Read the model definition and answer for the solid it produces. Units are mm, in the model's axes. A direction names the side the tool comes from. Coordinates: 2 decimals unless noted, no trailing zeros. Write each loop counter-clockwise with the first axis right and the second up, starting at its lowest first coordinate (ties: lowest second). Pieces come first, ordered by that corner, then holes. Notation, with made-up numbers: (88.25, 60) -> (97.25, 60) arc R11 cw to (97.25, 81) -> close; hole circle Ø8 at (78, -3). An arc over 180 degrees is marked (long way). Answer in a Markdown table with one row per item. Add a question column.
Item 1: Which of the six approach directions +Z, -Z, +X, -X, +Y, -Y give full straight-line access (tool end or side, diameter ignored) to faces 1 (the face through (19, 1, -11)), 2 (the face through (-12, 1, 19)), 3 (the face through (-12, 1, -19)), 4 (the face through (19, 1, 12)), 5 (the face through (2, 7, 46))?
Item 2: For a pull along X with two mould halves and no side action, classify faces 6 (the face through (4, 1, 34)), 7 (the face through (48, 11, 0)), 8 (the face through (44.391, 7.056, -0.028)), 9 (the face through (-4, 1, -34)) as +X half, -X half, draft (parallel to the pull), parting line (faces both ways), or undercut.
Item 3: Section C-C on y = 6.5 is taken. Count the separate pieces of the cut face and the enclosed holes in it, then the cut area to 3 significant figures.
Item 4: Straight lines are drawn through the part: line 1 (Z direction, x = -48, y = 2); line 2 (Y direction, x = 10, z = -17). For each, find the intervals that lie inside material, in ascending order. Write a range as from..to.
Item 5: Section A-A on x = 27.5 is taken. Write down the section's boundary in (y, z).
Item 6: Given pin 1 Ø12 at (x, z) = (0.5, -26) entering from +Y; pin 2 Ø1.1 at (x, y) = (48.5, 4) entering from +Z; pin 3 Ø1.1 at (y, z) = (4, -48.5) entering from +X; pin 4 Ø12 at (x, z) = (21, 25.5) entering from -Y, each flat-ended and moving along its own axis, determine where each tip first touches the part or whether it passes through.
Item 7: Section B-B on z = 16 is taken. Write down the section's boundary in (x, y).
```python
from build123d import *

# Parameters (mm, degrees)
SKETCH1_W           = 38
SKETCH1_H           = 38
BOSS_EXTRUDE1_DEPTH = 3
SKETCH2_W           = 30
SKETCH2_H           = 8
BOSS_EXTRUDE2_DEPTH = 3
SKETCH8_R           = 2.5
BOSS_EXTRUDE5_DEPTH = 2
CIRPATTERN1_COUNT   = 4


with BuildPart() as part:
    # Sketch1 → Boss-Extrude1 (new body)
    with BuildSketch(Plane(origin=(0, 0, 0), x_dir=(1, 0, 0), z_dir=(0, 1, 0))):
        Rectangle(SKETCH1_W, SKETCH1_H)
    extrude(amount=BOSS_EXTRUDE1_DEPTH)

    # Sketch2 → Boss-Extrude2 (add)
    with BuildSketch(Plane(origin=(0, 0, 0), x_dir=(1, 0, 0), z_dir=(0, 1, 0))):
        with Locations((-34, 0)):
            Rectangle(SKETCH2_W, SKETCH2_H)
    boss_extrude2 = extrude(amount=BOSS_EXTRUDE2_DEPTH)

    # Sweep1: sweep along a path in Sketch7
    with BuildLine(Plane.XY) as sweep1_path:
        Line((-46.5, 3), (-58.047005384, 23))
    # Sketch8 → Sweep1 (sweep)
    with BuildSketch(Plane(origin=(0, 3, 0), x_dir=(1, 0, 0), z_dir=(0, 1, 0))):
        with Locations((-46.5, 0)):
            Circle(SKETCH8_R)
    sweep1 = sweep(path=sweep1_path.line)

    # Sketch6 → Boss-Extrude5 (add, symmetric)
    with BuildSketch(Plane.XY):
        Polygon((-46.230461265, 11), (-42.5, 3), (-46.5, 3), (-49, 3), (-49, 11), align=None)
    boss_extrude5 = extrude(amount=BOSS_EXTRUDE5_DEPTH, both=True)

    # CirPattern1: Boss-Extrude2, Sweep1, Boss-Extrude5 ×4 about axis
    cirpattern1_axis = Axis((0, 0, 0), (0, 1, 0))
    for i in range(1, CIRPATTERN1_COUNT):
        add(boss_extrude2.rotate(cirpattern1_axis, i * 360 / CIRPATTERN1_COUNT))
        add(sweep1.rotate(cirpattern1_axis, i * 360 / CIRPATTERN1_COUNT))
        add(boss_extrude5.rotate(cirpattern1_axis, i * 360 / CIRPATTERN1_COUNT))


solid = part.part
```
Results below:
| question | item | result |
|---|---|---|
| 1 | face 1 | -Z, +X, +Y, -Y |
| 1 | face 2 | +Z, -X, +Y, -Y |
| 1 | face 3 | -Z, -X, +Y, -Y |
| 1 | face 4 | +Z, +X, +Y, -Y |
| 1 | face 5 | +X, +Y |
| 2 | face 6 | +X half |
| 2 | face 7 | undercut |
| 2 | face 8 | undercut |
| 2 | face 9 | -X half |
| 3 | separate pieces | 4 |
| 3 | enclosed holes | 0 |
| 3 | area | 114 mm2 |
| 4 | line 1 | z = -4..4 |
| 4 | line 2 | y = 0..3 |
| 5 | outline | (0, -4) -> (3, -4) -> (3, 4) -> (0, 4) -> close |
| 6 | pin 1 | stops at y = 3 |
| 6 | pin 2 | stops at z = 2.37 |
| 6 | pin 3 | stops at x = 2.37 |
| 6 | pin 4 | passes through |
| 7 | outline | (-19, 0) -> (19, 0) -> (19, 3) -> (-19, 3) -> close |
